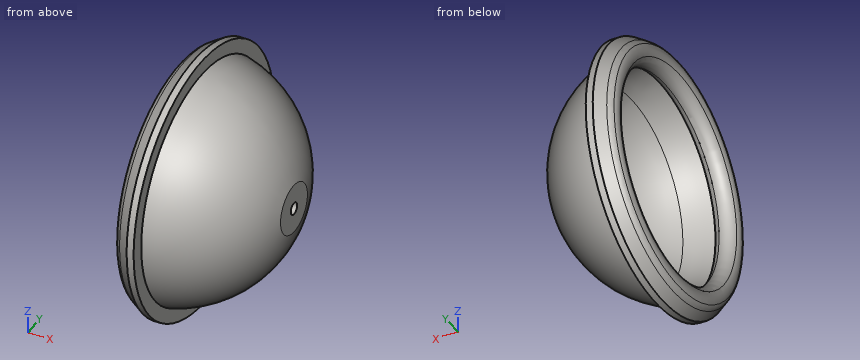
from build123d import *

# Parameters (mm, degrees)
F3_R     = 3.175
F4_DEPTH = 25.4
F3_R_2   = 13.462
F5_DEPTH = 9.017


with BuildPart() as f1:
    # F0 (on Front) → F1 (revolve)
    with BuildSketch(Plane.XZ):
        with BuildLine():
            Line((57.15, 0), (63.5, 0))
            ThreePointArc((63.5, 0), (49.7246437823, 39.4931614425), (14.3752818669, 61.8514451832))
            ThreePointArc((14.3752818669, 61.8514451832), (14.545447186, 61.0073776147), (14.6025029863, 60.1482205093))
            ThreePointArc((14.6025029863, 60.1482205093), (14.1437492907, 57.7501426695), (12.8322714456, 55.6907111604))
            ThreePointArc((12.8322714456, 55.6907111604), (20.1907637916, 53.46452616), (27.1838868177, 50.270854354))
            ThreePointArc((27.1838868177, 50.270854354), (49.0901295152, 29.2622911643), (57.15, 0))
        make_face()
        with BuildLine():
            ThreePointArc((14.6025029863, 60.1482205093), (14.545447186, 61.0073776147), (14.3752818669, 61.8514451832))
            ThreePointArc((14.3752818669, 61.8514451832), (8.4803191689, 62.9311861226), (2.5098197969, 63.4503806497))
            ThreePointArc((2.5098197969, 63.4503806497), (1.6097384582, 60.2943080474), (2.3670190255, 57.1009607707))
            ThreePointArc((2.3670190255, 57.1009607707), (7.632287252, 56.6380675103), (12.8322714456, 55.6907111604))
            ThreePointArc((12.8322714456, 55.6907111604), (14.1437492907, 57.7501426695), (14.6025029863, 60.1482205093))
        make_face()
        with BuildLine():
            ThreePointArc((12.8322714456, 55.6907111604), (7.632287252, 56.6380675103), (2.3670190255, 57.1009607707))
            ThreePointArc((2.3670190255, 57.1009607707), (5.5979999661, 54.1542983084), (9.9647443416, 53.9227792702))
            ThreePointArc((9.9647443416, 53.9227792702), (11.5150820885, 54.6176657234), (12.8322714456, 55.6907111604))
        make_face()
        with BuildLine():
            ThreePointArc((5.0834796416, 65.8999384363), (10.7005286229, 66.1045985568), (14.3752818669, 61.8514451832))
            Line((14.3752818669, 61.8514451832), (14.3752818669, 69.3246647716))
            Line((14.3752818669, 69.3246647716), (10.6675541028, 69.3246647716))
            Line((10.6675541028, 69.3246647716), (5.0834796416, 65.8999384363))
        make_face()
        with BuildLine():
            ThreePointArc((2.5098197969, 63.4503806497), (8.4803191689, 62.9311861226), (14.3752818669, 61.8514451832))
            ThreePointArc((14.3752818669, 61.8514451832), (10.7005286229, 66.1045985568), (5.0834796416, 65.8999384363))
            ThreePointArc((5.0834796416, 65.8999384363), (3.6259528632, 64.8545044217), (2.5098197969, 63.4503806497))
        make_face()
    revolve(axis=Axis((31.75, 0, 0), (1, 0, 0)))

    # F3 (on offset) → F4 (cut)
    with BuildSketch(Plane.YZ.offset(71.12)):
        Circle(F3_R)
    extrude(amount=-F4_DEPTH, mode=Mode.SUBTRACT)

    # F3 (on offset) → F5 (cut)
    with BuildSketch(Plane.YZ.offset(71.12)):
        Circle(F3_R_2)
        Circle(F3_R, mode=Mode.SUBTRACT)
    extrude(amount=-F5_DEPTH, mode=Mode.SUBTRACT)


solid = f1.part
Source: CAD feature listing. Evaluate the final solid. Frame: model axes, mm. Coordinates: 2 decimals unless noted, no trailing zeros. Loops run counter-clockwise (first coordinate to the right, second up) from the corner with the lowest first, then second, coordinate; pieces in that order, holes last. Notation, with made-up numbers: (58.5, -16) -> (67.5, -16) arc R34 ccw to (67.5, 14) -> close; hole circle Ø11 at (-6, 17). An arc over 180 degrees is marked (long way). Answer in a Markdown table with one row per item. Add a question column.
Q1. Ray query, line 1 along Z through (x, y) = (34.5, 18); line 2 along Y through (x, z) = (58.55, 0) (3 decimals); line 3 along Y through (x, z) = (59, 0) (3 decimals). Return the intervals inside material, ascending.
Q2. Section A-A on x = 43. Return the cut outline in (y, z), and give its area (3 significant figures).
Q3. Contact query for flat-ended pins moving along their axis: pin 1 Ø1 at (x, z) = (29.5, -32.5) entering from -Y; pin 2 Ø3 at (y, z) = (-27.5, -30) entering from -X; pin 3 Ø1 at (x, z) = (29.5, -34) entering from +Y; pin 4 Ø5 at (x, z) = (53, -42) entering from -Y. Output: stop coordinate, or through.
Computed values:
| question | item | result |
|---|---|---|
| 1 | line 1 | z = -50.18 to -41.86, 41.86 to 50.18 |
| 1 | line 2 | y = -24.579 to -3.175, 3.175 to 24.579 |
| 1 | line 3 | y = -23.479 to -3.175, 3.175 to 23.479 |
| 2 | outline | circle Ø93.45 at (0, 0); hole circle Ø75.29 at (0, 0) |
| 2 | area | 2,410 mm^2 |
| 3 | pin 1 | stops at y = -46.36 |
| 3 | pin 2 | stops at x = 38.54 |
| 3 | pin 3 | stops at y = 45.29 |
| 3 | pin 4 | passes through |
